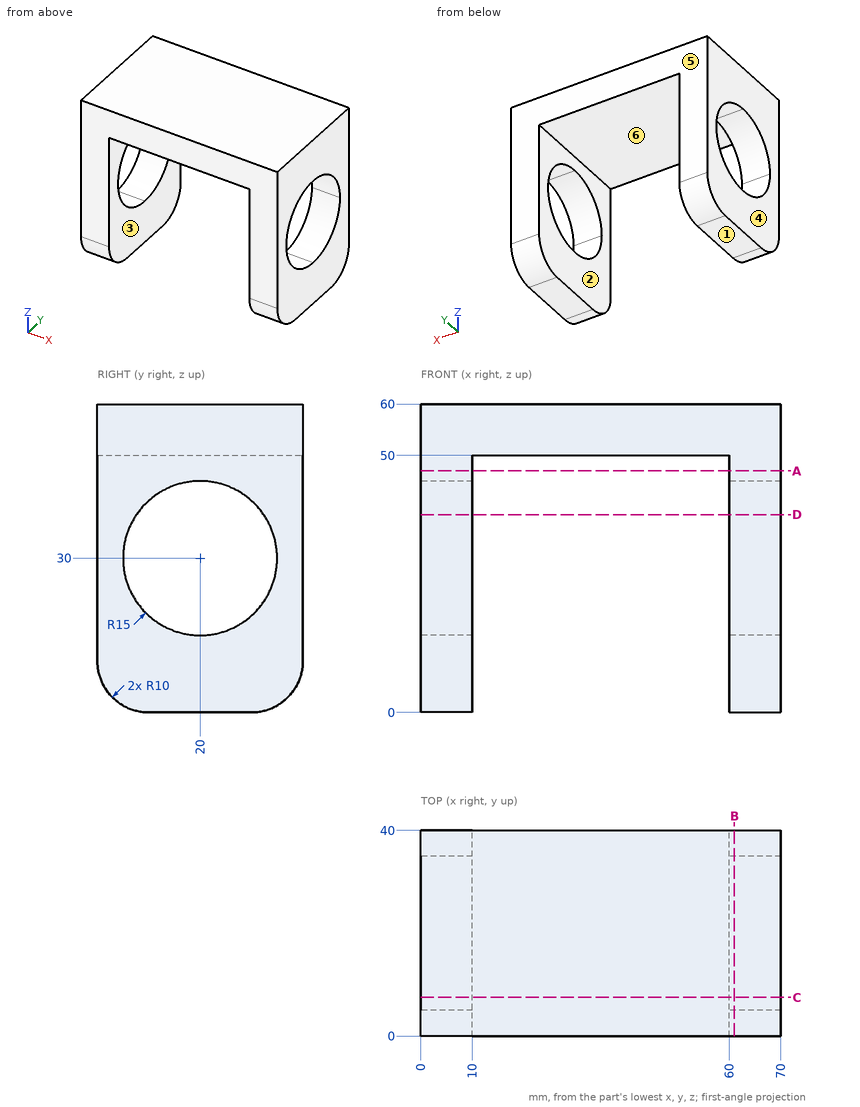
For this review, use the dimensioned drawing (mm, ordinates from the lowest corner) and the shaded views. A direction names the side the tool comes from. Give positions to 0.01 mm unless a question says otherwise; leave off trailing zeros. Order: outer loops, then holes, each group sorted by start corner. A loop starts at its lowest first (then second) coordinate and runs counter-clockwise, first axis right, second up. Notation, with made-up numbers: (-27.75, -15) - (-23.75, -15) arc R14 cw to (-23.75, -6) - close; hole circle Ø1 at (40, 38.5). An arc over 180 degrees is marked (long way). Use CSV: the item, a comma, the result in double quotes. Start each with the question number.
Q1. We need section A-A, the plane z = 47. Write out the cut boundary in (x, y).
Q2. To check wall thickness, follow line 1 along X through (y, z) = (28, 4); line 2 along Z through (x, y) = (53.5, 33.5); line 3 along Z through (x, y) = (63, 10.5). State the ranges of each line that lie inside material, in increasing order. Write a range as [from, to].
Q3. Clearance check with flat-ended pins moving along their axes: pin 1 Ø3 at (x, y) = (33, 29) entering from -Z; pin 2 Ø1 at (x, y) = (60, 4) entering from -Z. State where each tip first meets the part, or that it passes through.
Q4. We need section B-B, the plane x = 61. Write out the cut boundary in (y, z).
Q5. We need section C-C, the plane y = 7.5. Write out the cut boundary in (x, z), and give its area (3 significant figures).
Q6. We need section D-D, the plane z = 38.5. Write out the cut boundary in (x, y).
Q7. Tool access review of the marked faces 5 and 6: name each direction out of +Z, -Z, +X, -X, +Y, -Y from which nothing blocks a thin tool from reaching the whole face with its end or side.
Q8. The part is to be moulded in two halves that separate along X. For the marked faces 1, 2, 3 and 4, say which applies: +X half, -X half, draft (parallel to the pull), parting line (faces both ways), or undercut.
Outcome:
1,outline,"(0, 0) - (10, 0) - (10, 40) - (0, 40) - close; (60, 0) - (70, 0) - (70, 40) - (60, 40) - close"
2,line 1,"x = [0, 10], [60, 70]"
2,line 2,"z = [50, 60]"
2,line 3,"z = [0, 18.39], [41.61, 60]"
3,pin 1,"stops at z = 50"
3,pin 2,"stops at z = 1.65"
4,outline,"(0, 10) arc R10 ccw to (10, 0) - (30, 0) arc R10 ccw to (40, 10) - (40, 60) - (0, 60) - close; hole circle Ø30 at (20, 30)"
5,outline,"(0, 0.32) - (10, 0.32) - (10, 21.71) - (0, 21.71) - close; (0, 38.29) - (10, 38.29) - (10, 50) - (60, 50) - (60, 38.29) - (70, 38.29) - (70, 60) - (0, 60) - close; (60, 0.32) - (70, 0.32) - (70, 21.71) - (60, 21.71) - close"
5,area,"1,360 mm^2"
6,outline,"(0, 0) - (10, 0) - (10, 7.64) - (0, 7.64) - close; (0, 32.36) - (10, 32.36) - (10, 40) - (0, 40) - close; (60, 0) - (70, 0) - (70, 7.64) - (60, 7.64) - close; (60, 32.36) - (70, 32.36) - (70, 40) - (60, 40) - close"
7,face 5,"+Z, -Z, +X, -X, +Y"
7,face 6,"-Z, +Y, -Y"
8,face 1,"draft"
8,face 2,"undercut"
8,face 3,"undercut"
8,face 4,"-X half"
